from build123d import *

# Parameters (mm, degrees)
SKETCH2_W                    = 12.3776613
SKETCH2_H                    = 44.1706
F_3_8_16_TAPPED_HOLE2_REACH  = 91.671
F_3_8_16_TAPPED_HOLE2_BORE_R = 3.96875
CIRPATTERN1_COUNT            = 6


with BuildPart() as part:
    # Sketch2 → Revolve1 (revolve)
    with BuildSketch(Plane.XY, mode=Mode.PRIVATE) as revolve1_sk:
        with Locations((-28.71076935, 22.0853)):
            Rectangle(SKETCH2_W, SKETCH2_H)
    revolve(revolve1_sk.sketch.rotate(Axis((0, 0, 0), (0, 1, 0)), 270), axis=Axis((0, 0, 0), (0, 1, 0)))

    # 3/8-16 Tapped Hole2 bore → 3/8-16 Tapped Hole2 (cut, up to next)
    with BuildSketch(Plane(origin=(34.8996, 0, 0), x_dir=(0, 0, -1), z_dir=(1, 0, 0)), mode=Mode.PRIVATE) as f_3_8_16_tapped_hole2_sk1:
        with Locations((0, 24.4856)):
            Circle(F_3_8_16_TAPPED_HOLE2_BORE_R)
    f_3_8_16_tapped_hole2_tool1 = extrude(f_3_8_16_tapped_hole2_sk1.sketch, amount=-F_3_8_16_TAPPED_HOLE2_REACH, mode=Mode.PRIVATE) & part.part
    f_3_8_16_tapped_hole2 = f_3_8_16_tapped_hole2_tool1.solids().sort_by_distance((34.8996, 24.4856, 0))[0]
    add(f_3_8_16_tapped_hole2, mode=Mode.SUBTRACT)

    # CirPattern1: 3/8-16 Tapped Hole2 ×6 about axis
    cirpattern1_axis = Axis((0, 44.1706, 0), (0, -1, 0))
    for i in range(1, CIRPATTERN1_COUNT):
        add(f_3_8_16_tapped_hole2.rotate(cirpattern1_axis, i * 360 / CIRPATTERN1_COUNT), mode=Mode.SUBTRACT)


solid = part.part
Work out the finished part from the listing and answer in its coordinate system (mm). Give positions to 0.01 mm unless a question says otherwise; leave off trailing zeros. Loops run counter-clockwise (first coordinate to the right, second up) from the corner with the lowest first, then second, coordinate; pieces in that order, holes last. Notation, with made-up numbers: (23.5, 73.5) - (38.5, 73.5) arc R19 cw to (38.5, 106.5) - close; hole circle Ø6 at (51.5, -34). An arc over 180 degrees is marked (long way). Answer in a Markdown table with one row per item. Add a question column.
Q1. Determine the mould class of faces 1 (the flat face through (23, 0, 0)), 2 (the cylindrical face through (-13.57, 20.61, -25.22)), 3 (the cylindrical face through (21.986, 22.394, 4.882)), 4 (the cylindrical face through (30.962, 22.394, -16.104)) for opening direction Z: released by +Z, released by -Z, zero draft, split by the parting line, or undercut.
Q2. The part is cut by section D-D (z = 9.5). Determine the outline of the cut face in (x, y).
Q3. The part is cut by section B-B (x = 0). Determine the outline of the cut face in (y, z), and give its area (3 significant figures).
Q4. The part is cut by section C-C (y = 23.5). Determine the outline of the cut face in (x, z).
Q5. The part is cut by section A-A (z = 0). Determine the outline of the cut face in (x, y).
Q6. Each of these flat-tipped pins is pushed along its axis until it touches: P1, Ø5, axis at x = -15.5, y = 37.5, coming from the +Z side; P2, Ø12, axis at y = 18.5, z = -25, coming from the -X side; P3, Ø10, axis at y = 18.5, z = 5.5, coming from the -X side; P4, Ø6.5, axis at y = 24.49, z = 0, coming from the +X side. Where does it stop, or does it pass through?
Q7. Consider line 1 along X through (y, z) = (31, 0); line 2 along Y through (x, z) = (-31, 0); line 3 along Z through (x, y) = (-14, 31.5). Determine where each line is inside the solid, lowest interval first.
Solution:
| question | item | result |
|---|---|---|
| 1 | face 1 | zero draft |
| 1 | face 2 | undercut |
| 1 | face 3 | undercut |
| 1 | face 4 | split by the parting line |
| 2 | outline | (-33.58, 0) - (-20.42, 0) - (-20.42, 44.17) - (-33.58, 44.17) - close; (20.42, 0) - (33.58, 0) - (33.58, 44.17) - (20.42, 44.17) - close |
| 3 | outline | (0, -34.9) - (44.17, -34.9) - (44.17, -22.52) - (0, -22.52) - close; (0, 22.52) - (44.17, 22.52) - (44.17, 34.9) - (0, 34.9) - close |
| 3 | area | 1,090 mm² |
| 4 | outline | (-34.69, -3.84) arc R34.9 ccw to (-20.67, -28.12) - (-14.43, -17.3) arc R22.52 cw to (-22.19, -3.84) - close; (-34.69, 3.84) - (-22.19, 3.84) arc R22.52 cw to (-14.43, 17.3) - (-20.67, 28.12) arc R34.9 ccw to start; (-14.01, -31.96) arc R34.9 ccw to (14.01, -31.96) - (7.77, -21.14) arc R22.52 cw to (-7.77, -21.14) - close; (-14.01, 31.96) - (-7.77, 21.14) arc R22.52 cw to (7.77, 21.14) - (14.01, 31.96) arc R34.9 ccw to start; (14.43, -17.3) - (20.67, -28.12) arc R34.9 ccw to (34.69, -3.84) - (22.19, -3.84) arc R22.52 cw to start; (14.43, 17.3) arc R22.52 cw to (22.19, 3.84) - (34.69, 3.84) arc R34.9 ccw to (20.67, 28.12) - close |
| 5 | outline | (-34.9, 0) - (-22.52, 0) - (-22.52, 20.52) - (-34.9, 20.52) - close; (-34.9, 28.45) - (-22.52, 28.45) - (-22.52, 44.17) - (-34.9, 44.17) - close; (22.52, 0) - (34.9, 0) - (34.9, 20.52) - (22.52, 20.52) - close; (22.52, 28.45) - (34.9, 28.45) - (34.9, 44.17) - (22.52, 44.17) - close |
| 6 | P1 | stops at z = 32.39 |
| 6 | P2 | stops at x = -29.27 |
| 6 | P3 | stops at x = -34.9 |
| 6 | P4 | passes through |
| 7 | line 1 | x = -34.9 to -22.52, 22.52 to 34.9 |
| 7 | line 2 | y = 0 to 20.52, 28.45 to 44.17 |
| 7 | line 3 | z = -31.97 to -17.64, 17.64 to 31.97 |
